Model file for the job. Use its own axes, mm. Round coordinates to 2 decimals unless told otherwise and drop trailing zeros. Put each result on its own line as item: value. Start each with the question number.
Item 1: Probe probe 1 along Y at (x, z) = (-10, 252.5); probe 2 along Y at (x, z) = (5.5, 285); probe 3 along X at (y, z) = (3.75, 211.5). List the from-to ranges inside material, lowest first.
Item 2: Pin check, flat tips, straight feed: pin 1 Ø3.5 at (x, y) = (10, 10) entering from -Z; pin 2 Ø1.2 at (x, z) = (0, 235.5) entering from +Y; pin 3 Ø3 at (x, z) = (0, 282) entering from -Y; pin 4 Ø3 at (x, z) = (-1.5, 308) entering from -Y. Stop position of each tip, or through.
Item 3: Saw through at A-A on z = 29.5. State how many separate pieces and enclosed holes the cut face has, plus the area to 3 significant figures.
```python
from build123d import *

# Parameters (mm, degrees)
SKETCH1_R           = 2.5
SKETCH1_R_2         = 3
BOSS_EXTRUDE1_DEPTH = 400


with BuildPart() as part:
    # Sketch1 → Boss-Extrude1 (new body)
    with BuildSketch(Plane.XY):
        Polygon((-15, 15), (-3.35, 15), (-3.35, 12.901975832), (-6.216494866, 12.901975832), (-6.216494866, 8.323198212), (-2.018681454, 4.1253848), (2.018681454, 4.1253848), (6.216494866, 8.323198212), (6.216494866, 12.901975832), (3.35, 12.901975832), (3.35, 15), (15, 15), (15, 3.35), (12.901975832, 3.35), (12.901975832, 6.216494866), (8.323198212, 6.216494866), (4.1253848, 2.018681454), (4.1253848, -2.018681454), (8.323198212, -6.216494866), (12.901975832, -6.216494866), (12.901975832, -3.35), (15, -3.35), (15, -15), (3.35, -15), (3.35, -12.901975832), (6.216494866, -12.901975832), (6.216494866, -8.323198212), (2.018681454, -4.1253848), (-2.018681454, -4.1253848), (-6.216494866, -8.323198212), (-6.216494866, -12.901975832), (-3.35, -12.901975832), (-3.35, -15), (-15, -15), (-15, -3.35), (-12.901975832, -3.35), (-12.901975832, -6.216494866), (-8.323198212, -6.216494866), (-4.1253848, -2.018681454), (-4.1253848, 2.018681454), (-8.323198212, 6.216494866), (-12.901975832, 6.216494866), (-12.901975832, 3.35), (-15, 3.35), align=None)
        Circle(SKETCH1_R, mode=Mode.SUBTRACT)
        with Locations((10, 10)):
            Circle(SKETCH1_R_2, mode=Mode.SUBTRACT)
        with Locations((-10, 10)):
            Circle(SKETCH1_R_2, mode=Mode.SUBTRACT)
        with Locations((-10, -10)):
            Circle(SKETCH1_R_2, mode=Mode.SUBTRACT)
        with Locations((10, -10)):
            Circle(SKETCH1_R_2, mode=Mode.SUBTRACT)
    extrude(amount=BOSS_EXTRUDE1_DEPTH)


solid = part.part
```
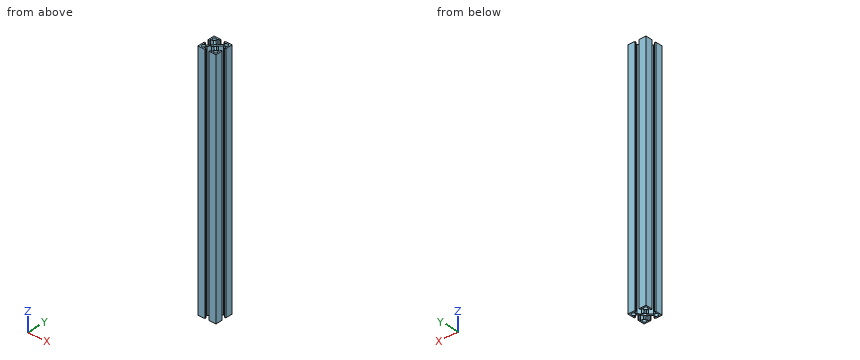
Results found:
1. probe 1: y = -15 to -13, -7 to -6.22, 6.22 to 7, 13 to 15
1. probe 2: y = -15 to -12.9, -7.61 to -3.39, 3.39 to 7.61, 12.9 to 15
1. probe 3: x = -15 to -12.9, -5.86 to 5.86, 12.9 to 15
2. pin 1: passes through
2. pin 2: stops at y = 4.13
2. pin 3: stops at y = -4.13
2. pin 4: stops at y = -5.11
3. separate pieces: 1
3. enclosed holes: 5
3. area: 345 mm²
